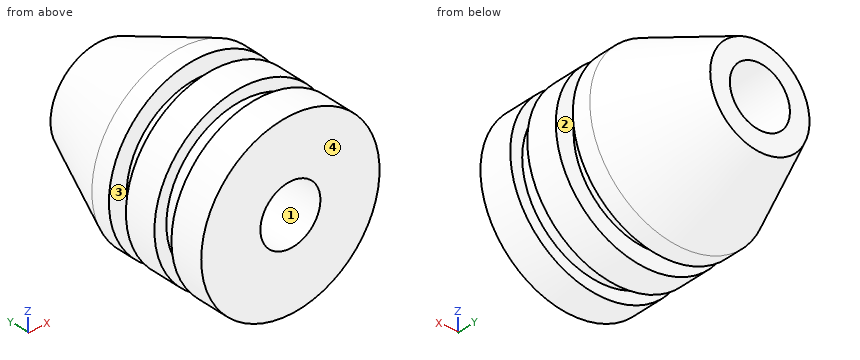
Autodesk Inventor part; units mm, degrees
ref_plane "Work Plane1" through (0, 44.7, 0) normal (0, 1, 0) x (1, 0, 0)
ref_plane "YZ Plane" through (0, 0, 0) normal (1, 0, 0) x (0, 1, 0)
ref_plane "XZ Plane" through (0, 0, 0) normal (0, 1, 0) x (-1, 0, 0)
sketch "Sketch1" plane through (0, 0, 0) normal (0, 1, 0) x (-1, 0, 0)
  circle A0 centre (0, 0) radius 18.85
  dimension "d0" = 37.7
extrude "Extrusion1" add sketch "Sketch1" along normal blind 7
sketch "Sketch2" plane through (0, 7, 0) normal (0, 1, 0) x (1, 0, 0)
  circle A0 centre (0, 0) radius 16.325
  dimension "d3" = 32.65
extrude "Extrusion2" add sketch "Sketch2" along normal blind 4
sketch "Sketch3" plane through (0, 11, 0) normal (0, 1, 0) x (1, 0, 0)
  circle A0 centre (0, 0) radius 18.85
  dimension "d6" = 37.7
extrude "Extrusion3" add sketch "Sketch3" along normal blind 6.7
sketch "Sketch4" plane through (0, 17.7, 0) normal (0, 1, 0) x (1, 0, 0)
  circle A0 centre (0, 0) radius 15.1
  dimension "d9" = 30.2
extrude "Extrusion4" add sketch "Sketch4" along normal blind 4
sketch "Sketch5" plane through (0, 21.7, 0) normal (0, 1, 0) x (1, 0, 0)
  circle A0 centre (0, 0) radius 18.85
  dimension "d12" = 37.7
extrude "Extrusion5" add sketch "Sketch5" along normal blind 4
ref_plane "Work Plane1" through (0, 44.7, 0) normal (0, 1, 0) x (1, 0, 0)
sketch "Sketch6" plane through (0, 44.7, 0) normal (0, 1, 0) x (1, 0, 0)
  circle A0 centre (0, 0) radius 10.5
  dimension "d16" = 21
loft "Loft1" add profiles "Sketch6" section 2 edges at (-18.85, 25.7, 0)
sketch "Sketch7" plane through (0, 44.7, 0) normal (0, 1, 0) x (1, 0, 0)
  circle A0 centre (0, 0) radius 6.35
  dimension "d21" = 12.7
extrude "Extrusion6" cut sketch "Sketch7" against normal through all
properties part number "Soporte Intermedio" material "Steel, Alloy"
Geometry: final body of the model. Coordinates: model frame, mm. Face numbers are marked on the shaded views. Coordinates: 2 decimals unless noted, no trailing zeros. Order: outer loops, then holes, each group sorted by start corner. A loop starts at its lowest first (then second) coordinate and runs counter-clockwise, first axis right, second up. Notation, with made-up numbers: (32.25, 38) -> (45.25, 38) arc R26 cw to (45.25, 66) -> close; hole circle Ø7 at (-26, 74). An arc over 180 degrees is marked (long way). Write each question's results on one line, items separated by ' | '. Start each with the question number.
1) Cut plane B-B, the plane y = 14. Output: boundary loops of the cut face in (x, z), and give its area (3 significant figures).
2) First-contact query: pin 1 (19 mm diameter, centred on x = -5.5, z = -6.5, fed in from -Y); pin 2 (12 mm diameter, centred on x = 12, y = 29, fed in from -Z); pin 3 (8 mm diameter, centred on y = 25.5, z = 12.5, fed in from -X); pin 4 (2 mm diameter, centred on y = 11.5, z = -6.5, fed in from -X). Flat tips, straight axial feed; report the tip coordinate or a pass-through.
3) Mould query, pull axis Y, two halves, no side actions, for the marked faces 1, 2, 3 and 4. Classes: released by +Y, released by -Y, zero draft, split by the parting line, or undercut.
4) Cut plane A-A, the plane x = 0. Output: boundary loops of the cut face in (y, z) (3 decimals), and give its area (3 significant figures).
5) Material intervals for line 1 along Y through (x, z) = (-11, 13); line 2 along X through (y, z) = (18, 0); line 3 along Z through (x, y) = (0, 9) (3 decimals), sorted ascending.
6) Cut plane C-C, the plane y = 9. Output: boundary loops of the cut face in (x, z) (3 decimals), and give its area (3 significant figures).
Checks:
1) outline: circle Ø37.7 at (0, 0); hole circle Ø12.7 at (0, 0) | area: 990 mm^2
2) pin 1: y = 0 | pin 2: z = -17.51 | pin 3: x = -16.82 | pin 4: x = -18.03
3) face 1: zero draft | face 2: undercut | face 3: undercut | face 4: released by -Y
4) outline: (0, -18.85) -> (7, -18.85) -> (7, -16.325) -> (11, -16.325) -> (11, -18.85) -> (17.7, -18.85) -> (17.7, -15.1) -> (21.7, -15.1) -> (21.7, -18.85) -> (25.7, -18.85) -> (44.7, -10.5) -> (44.7, -6.35) -> (0, -6.35) -> close; (0, 6.35) -> (44.7, 6.35) -> (44.7, 10.5) -> (25.7, 18.85) -> (21.7, 18.85) -> (21.7, 15.1) -> (17.7, 15.1) -> (17.7, 18.85) -> (11, 18.85) -> (11, 16.325) -> (7, 16.325) -> (7, 18.85) -> (0, 18.85) -> close | area: 909 mm^2
5) line 1: 0 to 7, 11 to 17.7, 21.7 to 29.84 | line 2: -15.1 to -6.35, 6.35 to 15.1 | line 3: -16.325 to -6.35, 6.35 to 16.325
6) outline: circle Ø32.65 at (0, 0); hole circle Ø12.7 at (0, 0) | area: 711 mm^2
